For this review, take the finished solid that the model builds, in its own axes (mm). Coordinates: 2 decimals unless noted, no trailing zeros. Loops run counter-clockwise (first coordinate to the right, second up) from the corner with the lowest first, then second, coordinate; pieces in that order, holes last. Notation, with made-up numbers: (-27.5, 31.5) -> (20.5, 31.5) arc R30 cw to (20.5, 66.5) -> close; hole circle Ø11 at (-17.5, -23.5). An arc over 180 degrees is marked (long way). Use a Markdown table: item, result.
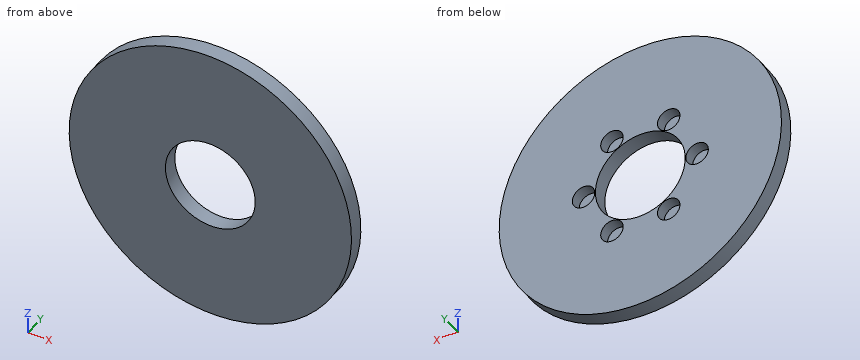
from build123d import *

# Parameters (mm, degrees)
SKETCH1_R             = 55
BOSS_EXTRUDE1_DEPTH   = 6
SKETCH2_R             = 17.5
CUT_EXTRUDE1_DEPTH    = 79.012819459
SKETCH3_R             = 4.37630442
CUT_EXTRUDE2_DEPTH    = 4.409124
CIRPATTERN1_START     = 1.590875617
CIRPATTERN1_OUTLINE_R = 4.37630442
CIRPATTERN1_DEPTH     = 4.409124383


# Read off the part's stored shape, not the designer's step: CirPattern1
with BuildPart() as part:
    # Sketch1 → Boss-Extrude1 (new body)
    with BuildSketch(Plane(origin=(0, 0, 0), x_dir=(1, 0, 0), z_dir=(0, 1, 0))):
        with Locations(Location((0, 0, 0), (0, 0, 270))):
            Circle(SKETCH1_R)
    extrude(amount=BOSS_EXTRUDE1_DEPTH)

    # Sketch2 → Cut-Extrude1 (cut, through all)
    with BuildSketch(Plane(origin=(0, 0, 0), x_dir=(1, 0, 0), z_dir=(0, 1, 0))):
        with Locations(Location((0, 0, 0), (0, 0, 270))):
            Circle(SKETCH2_R)
    extrude(amount=CUT_EXTRUDE1_DEPTH, mode=Mode.SUBTRACT)

    # Sketch3 → Cut-Extrude2 (cut)
    with BuildSketch(Plane(origin=(0, 6, 0), x_dir=(1, 0, 0), z_dir=(0, 1, 0))):
        with Locations(Location((-22.122792646, 0, 0), (0, 0, 270))):
            Circle(SKETCH3_R)
    extrude(amount=-CUT_EXTRUDE2_DEPTH, mode=Mode.SUBTRACT)

    # CirPattern1 outline → CirPattern1 (cut)
    with BuildSketch(Plane(origin=(0, 0, 0), x_dir=(1, 0, 0), z_dir=(0, 1, 0)).offset(CIRPATTERN1_START)):
        with Locations((-11.061396323, -19.158900434)):
            Circle(CIRPATTERN1_OUTLINE_R)
        with Locations((11.061396323, -19.158900434)):
            Circle(CIRPATTERN1_OUTLINE_R)
        with Locations((22.122792646, 0)):
            Circle(CIRPATTERN1_OUTLINE_R)
        with Locations((11.061396323, 19.158900434)):
            Circle(CIRPATTERN1_OUTLINE_R)
        with Locations((-11.061396323, 19.158900434)):
            Circle(CIRPATTERN1_OUTLINE_R)
    extrude(amount=CIRPATTERN1_DEPTH, mode=Mode.SUBTRACT)


solid = part.part
(1) Take a section at C-C on y = 3.8. Write out the cut boundary in (x, z).
Found:
| item | result |
|---|---|
| outline | circle Ø110 at (0, 0); hole circle Ø8.75 at (-22.12, 0); hole circle Ø35 at (0, 0); hole circle Ø8.75 at (-11.06, -19.16); hole circle Ø8.75 at (-11.06, 19.16); hole circle Ø8.75 at (11.06, -19.16); hole circle Ø8.75 at (11.06, 19.16); hole circle Ø8.75 at (22.12, 0) |
(2) For line 1 along X through (y, z) = (2.45, 0); line 2 along X through (y, z) = (4.45, -3); line 3 along Z through (x, y) = (-6.5, 1.2), list the stretches that pass through material, from the lowest coordinate up.
Found:
| item | result |
|---|---|
| line 1 | x = -55 to -26.5, -17.75 to -17.5, 17.5 to 17.75, 26.5 to 55 |
| line 2 | x = -54.92 to -25.31, -18.94 to -17.24, 17.24 to 18.94, 25.31 to 54.92 |
| line 3 | z = -54.61 to -16.25, 16.25 to 54.61 |
(3) Take a section at B-B on x = 0. Write out the cut boundary in (y, z).
Found:
| item | result |
|---|---|
| outline | (0, -55) -> (6, -55) -> (6, -17.5) -> (0, -17.5) -> close; (0, 17.5) -> (6, 17.5) -> (6, 55) -> (0, 55) -> close |
(4) Take a section at A-A on z = 0. Write out the cut boundary in (x, y).
Found:
| item | result |
|---|---|
| outline | (-55, 0) -> (-17.5, 0) -> (-17.5, 6) -> (-17.75, 6) -> (-17.75, 1.59) -> (-26.5, 1.59) -> (-26.5, 6) -> (-55, 6) -> close; (17.5, 0) -> (55, 0) -> (55, 6) -> (26.5, 6) -> (26.5, 1.59) -> (17.75, 1.59) -> (17.75, 6) -> (17.5, 6) -> close |
(5) Take a section at D-D on x = -14. Write out the cut boundary in (y, z).
Found:
| item | result |
|---|---|
| outline | (0, -53.19) -> (6, -53.19) -> (6, -22.4) -> (1.59, -22.4) -> (1.59, -15.92) -> (6, -15.92) -> (6, -10.5) -> (0, -10.5) -> close; (0, 10.5) -> (6, 10.5) -> (6, 15.92) -> (1.59, 15.92) -> (1.59, 22.4) -> (6, 22.4) -> (6, 53.19) -> (0, 53.19) -> close |
(6) For pin 1 Ø5.5 at (x, z) = (11.06, -19.16) entering from +Y; pin 2 Ø1.5 at (x, y) = (-12.5, 3) entering from -Z; pin 3 Ø1 at (x, y) = (-19, 5) entering from +Z, all flat-tipped, find the tip position at first contact; note any pin that passes through.
Found:
| item | result |
|---|---|
| pin 1 | stops at y = 1.59 |
| pin 2 | stops at z = -53.73 |
| pin 3 | stops at z = 51.8 |
